Design review of the part built by this model. Coordinates are the model's own, in mm. Give positions to 0.01 mm unless a question says otherwise; leave off trailing zeros. Answer in a Markdown table with one row per item.
```python
from build123d import *

# Parameters (mm, degrees)
F0_R     = 7.6071600852
F1_DEPTH = 19.09754
F1_TAPER = -3


with BuildPart() as f1:
    # F0 (on Front) → F1 (new body)
    with BuildSketch(Plane.XZ):
        with BuildLine():
            ThreePointArc((-4.6388319141, 18.7061527472), (-1.4012654558, 19.2217420452), (1.8768469353, 19.1811458915))
            Line((1.8768469353, 19.1811458915), (8.2491056776, 22.2835490331))
            Line((8.2491056776, 22.2835490331), (0, 50.3449775279))
            Line((0, 50.3449775279), (-9.9238500669, 21.5898471936))
            Line((-9.9238500669, 21.5898471936), (-4.6388319141, 18.7061527472))
        make_face()
        with BuildLine():
            Line((9.9238500669, -21.5898471936), (4.6388319141, -18.7061527472))
            ThreePointArc((4.6388319141, -18.7061527472), (1.4012654558, -19.2217420452), (-1.8768469353, -19.1811458915))
            Line((-1.8768469353, -19.1811458915), (-8.2491056776, -22.2835490331))
            Line((-8.2491056776, -22.2835490331), (0, -50.3449775279))
            Line((0, -50.3449775279), (9.9238500669, -21.5898471936))
        make_face()
        with BuildLine():
            Line((-8.2491056776, -22.2835490331), (-1.8768469353, -19.1811458915))
            ThreePointArc((-1.8768469353, -19.1811458915), (-6.0612417477, -18.294815129), (-9.9470979542, -16.5073969607))
            Line((-9.9470979542, -16.5073969607), (-8.2491056776, -22.2835490331))
        make_face()
        with BuildLine():
            ThreePointArc((18.7061527472, 4.6388319141), (19.1305766639, 2.3366532985), (19.2727505076, 0))
            ThreePointArc((19.2727505076, 0), (19.2498357311, -0.9395405559), (19.1811458915, -1.8768469353))
            Line((19.1811458915, -1.8768469353), (22.2835490331, -8.2491056776))
            Line((22.2835490331, -8.2491056776), (50.3449775279, 0))
            Line((50.3449775279, 0), (21.5898471936, 9.9238500669))
            Line((21.5898471936, 9.9238500669), (18.7061527472, 4.6388319141))
        make_face()
        with BuildLine():
            Line((22.2835490331, -8.2491056776), (16.5073969607, -9.9470979542))
            ThreePointArc((16.5073969607, -9.9470979542), (14.5826684524, -12.6009798404), (12.2359871356, -14.890249526))
            Line((12.2359871356, -14.890249526), (9.9238500669, -21.5898471936))
            Line((9.9238500669, -21.5898471936), (35.5992750086, -35.5992750086))
            Line((35.5992750086, -35.5992750086), (22.2835490331, -8.2491056776))
        make_face()
        with BuildLine():
            ThreePointArc((14.890249526, 12.2359871356), (17.2223329805, 8.6504426961), (18.7061527472, 4.6388319141))
            Line((18.7061527472, 4.6388319141), (21.5898471936, 9.9238500669))
            Line((21.5898471936, 9.9238500669), (14.890249526, 12.2359871356))
        make_face()
        with BuildLine():
            ThreePointArc((1.8768469353, 19.1811458915), (6.0612417477, 18.294815129), (9.9470979542, 16.5073969607))
            Line((9.9470979542, 16.5073969607), (8.2491056776, 22.2835490331))
            Line((8.2491056776, 22.2835490331), (1.8768469353, 19.1811458915))
        make_face()
        with BuildLine():
            ThreePointArc((-19.1811458915, 1.8768469353), (-18.294815129, 6.0612417477), (-16.5073969607, 9.9470979542))
            Line((-16.5073969607, 9.9470979542), (-22.2835490331, 8.2491056776))
            Line((-22.2835490331, 8.2491056776), (-19.1811458915, 1.8768469353))
        make_face()
        with BuildLine():
            ThreePointArc((-12.2359871356, 14.890249526), (-8.6504426961, 17.2223329805), (-4.6388319141, 18.7061527472))
            Line((-4.6388319141, 18.7061527472), (-9.9238500669, 21.5898471936))
            Line((-9.9238500669, 21.5898471936), (-12.2359871356, 14.890249526))
        make_face()
        with BuildLine():
            Line((-21.5898471936, -9.9238500669), (-14.890249526, -12.2359871356))
            ThreePointArc((-14.890249526, -12.2359871356), (-17.2223329805, -8.6504426961), (-18.7061527472, -4.6388319141))
            Line((-18.7061527472, -4.6388319141), (-21.5898471936, -9.9238500669))
        make_face()
        with BuildLine():
            Line((9.9238500669, -21.5898471936), (12.2359871356, -14.890249526))
            ThreePointArc((12.2359871356, -14.890249526), (8.6504426961, -17.2223329805), (4.6388319141, -18.7061527472))
            Line((4.6388319141, -18.7061527472), (9.9238500669, -21.5898471936))
        make_face()
        with BuildLine():
            Line((22.2835490331, -8.2491056776), (19.1811458915, -1.8768469353))
            ThreePointArc((19.1811458915, -1.8768469353), (18.294815129, -6.0612417477), (16.5073969607, -9.9470979542))
            Line((16.5073969607, -9.9470979542), (22.2835490331, -8.2491056776))
        make_face()
        with BuildLine():
            ThreePointArc((9.9470979542, 16.5073969607), (12.6009798404, 14.5826684524), (14.890249526, 12.2359871356))
            Line((14.890249526, 12.2359871356), (21.5898471936, 9.9238500669))
            Line((21.5898471936, 9.9238500669), (35.5992750086, 35.5992750086))
            Line((35.5992750086, 35.5992750086), (8.2491056776, 22.2835490331))
            Line((8.2491056776, 22.2835490331), (9.9470979542, 16.5073969607))
        make_face()
        with BuildLine():
            ThreePointArc((-16.5073969607, 9.9470979542), (-14.5826684524, 12.6009798404), (-12.2359871356, 14.890249526))
            Line((-12.2359871356, 14.890249526), (-9.9238500669, 21.5898471936))
            Line((-9.9238500669, 21.5898471936), (-35.5992750086, 35.5992750086))
            Line((-35.5992750086, 35.5992750086), (-22.2835490331, 8.2491056776))
            Line((-22.2835490331, 8.2491056776), (-16.5073969607, 9.9470979542))
        make_face()
        with BuildLine():
            ThreePointArc((-18.7061527472, -4.6388319141), (-19.2217420452, -1.4012654558), (-19.1811458915, 1.8768469353))
            Line((-19.1811458915, 1.8768469353), (-22.2835490331, 8.2491056776))
            Line((-22.2835490331, 8.2491056776), (-50.3449775279, 0))
            Line((-50.3449775279, 0), (-21.5898471936, -9.9238500669))
            Line((-21.5898471936, -9.9238500669), (-18.7061527472, -4.6388319141))
        make_face()
        with BuildLine():
            Line((-8.2491056776, -22.2835490331), (-9.9470979542, -16.5073969607))
            ThreePointArc((-9.9470979542, -16.5073969607), (-12.6009798404, -14.5826684524), (-14.890249526, -12.2359871356))
            Line((-14.890249526, -12.2359871356), (-21.5898471936, -9.9238500669))
            Line((-21.5898471936, -9.9238500669), (-35.5992750086, -35.5992750086))
            Line((-35.5992750086, -35.5992750086), (-8.2491056776, -22.2835490331))
        make_face()
        with BuildLine():
            ThreePointArc((19.1811458915, -1.8768469353), (19.2498357311, -0.9395405559), (19.2727505076, 0))
            ThreePointArc((19.2727505076, 0), (19.1305766639, 2.3366532985), (18.7061527472, 4.6388319141))
            ThreePointArc((18.7061527472, 4.6388319141), (17.2223329805, 8.6504426961), (14.890249526, 12.2359871356))
            ThreePointArc((14.890249526, 12.2359871356), (12.6009798404, 14.5826684524), (9.9470979542, 16.5073969607))
            ThreePointArc((9.9470979542, 16.5073969607), (6.0612417477, 18.294815129), (1.8768469353, 19.1811458915))
            ThreePointArc((1.8768469353, 19.1811458915), (-1.4012654558, 19.2217420452), (-4.6388319141, 18.7061527472))
            ThreePointArc((-4.6388319141, 18.7061527472), (-8.6504426961, 17.2223329805), (-12.2359871356, 14.890249526))
            ThreePointArc((-12.2359871356, 14.890249526), (-14.5826684524, 12.6009798404), (-16.5073969607, 9.9470979542))
            ThreePointArc((-16.5073969607, 9.9470979542), (-18.294815129, 6.0612417477), (-19.1811458915, 1.8768469353))
            ThreePointArc((-19.1811458915, 1.8768469353), (-19.2217420452, -1.4012654558), (-18.7061527472, -4.6388319141))
            ThreePointArc((-18.7061527472, -4.6388319141), (-17.2223329805, -8.6504426961), (-14.890249526, -12.2359871356))
            ThreePointArc((-14.890249526, -12.2359871356), (-12.6009798404, -14.5826684524), (-9.9470979542, -16.5073969607))
            ThreePointArc((-9.9470979542, -16.5073969607), (-6.0612417477, -18.294815129), (-1.8768469353, -19.1811458915))
            ThreePointArc((-1.8768469353, -19.1811458915), (1.4012654558, -19.2217420452), (4.6388319141, -18.7061527472))
            ThreePointArc((4.6388319141, -18.7061527472), (8.6504426961, -17.2223329805), (12.2359871356, -14.890249526))
            ThreePointArc((12.2359871356, -14.890249526), (14.5826684524, -12.6009798404), (16.5073969607, -9.9470979542))
            ThreePointArc((16.5073969607, -9.9470979542), (18.294815129, -6.0612417477), (19.1811458915, -1.8768469353))
        make_face()
        Circle(F0_R, mode=Mode.SUBTRACT)
    extrude(amount=-F1_DEPTH, taper=F1_TAPER)


solid = f1.part
```
1) Add section A-A (x = -26). Count the separate pieces of the cut face and the enclosed holes in it, and give its area (3 significant figures).
Geometry says:
| item | result |
|---|---|
| separate pieces | 3 |
| enclosed holes | 0 |
| area | 904 mm^2 |
2) To check wall thickness, follow probe 1 along Z at (x, y) = (-28.5, 2); probe 2 along X at (y, z) = (17, -30.5); probe 3 along X at (y, z) = (5.75, -32). State the ranges of each line that lie inside material, in increasing order. Write a range as [from, to].
Geometry says:
| item | result |
|---|---|
| probe 1 | [-32.26, -22.37], [-7.65, 6.53], [20.78, 31.85] |
| probe 2 | [-33.83, -23.09], [-6.76, 7.79], [24.39, 34.11] |
| probe 3 | [-33.98, -27.52], [-5.71, 6.65], [28.37, 34.18] |
3) The part is to be moulded in two halves that separate along Z. For faces 1 (the face through (-7, 0, 4)), 2 (the face through (-5.634, 9.682, 4.32)), say which applies: released by +Z, released by -Z, zero draft, split by the parting line, or undercut.
Geometry says:
| item | result |
|---|---|
| face 1 | zero draft |
| face 2 | undercut |
4) Insertion check: P1, Ø1.5, axis at x = 39.5, y = 16.5, coming from the -Z side; P2, Ø8, axis at y = 8.5, z = 28.5, coming from the +X side; P3, Ø5, axis at x = 32.5, y = 8.5, coming from the -Z side. Each pin has a flat end and moves straight along its axis. Give the tip position at first contact, or say it passes through.
Geometry says:
| item | result |
|---|---|
| P1 | z = -4.31 |
| P2 | x = 34.43 |
| P3 | z = -35.79 |
